```python
from build123d import *

# Parameters (mm, degrees)
F0_W     = 22.7
F0_H     = 42
F1_DEPTH = 13.8
F3_DEPTH = 8.5
F5_DEPTH = 45.1
F7_DEPTH = 3


with BuildPart() as f1:
    # F0 (on Front) → F1 (new body)
    with BuildSketch(Plane.XZ):
        with Locations((0, -9.8)):
            Rectangle(F0_W, F0_H)
    extrude(amount=-F1_DEPTH)

    # F2 (on face) → F3 (join)
    with BuildSketch(Plane.XZ):
        with BuildLine():
            Line((1.966596, 1.85), (-1.966596, 1.85))
            ThreePointArc((-1.966596, 1.85), (-2.7, 0), (-1.966596, -1.85))
            Line((-1.966596, -1.85), (1.966596, -1.85))
            ThreePointArc((1.966596, -1.85), (2.7, 0), (1.966596, 1.85))
        make_face()
    extrude(amount=F3_DEPTH)

    # F4 (on face) → F5 (join)
    with BuildSketch(Plane.XZ):
        with BuildLine():
            Line((7.168159, -13.2), (-7.168159, -13.2))
            ThreePointArc((-7.168159, -13.2), (-11.35, -22), (-7.168159, -30.8))
            Line((-7.168159, -30.8), (7.168159, -30.8))
            ThreePointArc((7.168159, -30.8), (11.35, -22), (7.168159, -13.2))
        make_face()
    extrude(amount=-F5_DEPTH)

    # F6 (on Right) → F7 (join, symmetric)
    with BuildSketch(Plane.YZ):
        Polygon((21.067004, -7.2), (13.8, -7.2), (13.8, -36.8), (21.067004, -36.8), (21.067004, -32.191654), (45.1, -32.191654), (45.1, -11.808346), (21.067004, -11.808346), align=None)
    extrude(amount=F7_DEPTH, both=True)


solid = f1.part
```
CAD build for the part. Positions are in the model's coordinates, mm. A direction names the side the tool comes from. Coordinates: 2 decimals unless noted, no trailing zeros. Order: outer loops, then holes, each group sorted by start corner. A loop starts at its lowest first (then second) coordinate and runs counter-clockwise, first axis right, second up. Notation, with made-up numbers: M -25.5,24 L 17.5,24 A12 cw 17.5,28 Z; hole C 64.25,20.25 d7. An arc over 180 degrees is marked long. Write each question's results on one line, items separated by ' | '. Start each with the question number.
Q1. Which spindle directions (+Z, -Z, +X, -X, +Y, -Y) get a long thin tool onto all of the face, cutting with end or side? Do faces 1 (the flat face through (0, 17, -7.2)), 2 (the flat face through (3, 22, -12)), 3 (the flat face through (-3, 22, -12)). Say none if no direction does.
Q2. Cut at C-C (y = 28.5). List the corners of the cut face in (x, z).
Q3. Cut at A-A (x = 1). List the corners of the cut face in (y, z).
Q4. Cut at B-B (z = -9.5). List the corners of the cut face in (x, y).
Q5. Flat gauge pins, fed straight in: P1, Ø6, axis at x = 3, y = 16.5, coming from the +Z side; P2, Ø1, axis at x = -2, z = -11.5, coming from the -Y side; P3, Ø3.5, axis at x = 1, z = -9.5, coming from the +Y side; P4, Ø5, axis at x = -1.5, y = 26.5, coming from the -Z side. Where does each tip first touch, or does it go through?
Q6. Drill centre lines: probe 1 along Z at (x, y) = (1.5, -4); probe 2 along Y at (x, z) = (7.5, -19); probe 3 along Z at (x, y) = (8.5, 10). Where is each one in solid material? Low to high. Write a range as from..to.
Q7. Cut at D-D (y = 16.5). List the corners of the cut face in (x, z).
Found:
1) face 1: +Z, +X, -X, +Y | face 2: +Z, +X, +Y | face 3: +Z, -X, +Y
2) outline: M -7.17,-30.8 L -3,-30.8 L -3,-32.19 L 3,-32.19 L 3,-30.8 L 7.17,-30.8 A11.35 ccw 7.17,-13.2 L 3,-13.2 L 3,-11.81 L -3,-11.81 L -3,-13.2 L -7.17,-13.2 A11.35 ccw Z
3) outline: M -8.5,-1.85 L 0,-1.85 L 0,-30.8 L 13.8,-30.8 L 13.8,-36.8 L 21.07,-36.8 L 21.07,-32.19 L 45.1,-32.19 L 45.1,-11.81 L 21.07,-11.81 L 21.07,-7.2 L 13.8,-7.2 L 13.8,11.2 L 0,11.2 L 0,1.85 L -8.5,1.85 Z
4) outline: M -11.35,0 L 11.35,0 L 11.35,13.8 L 3,13.8 L 3,21.07 L -3,21.07 L -3,13.8 L -11.35,13.8 Z
5) P1: z = 11.2 | P2: y = 0 | P3: y = 21.07 | P4: z = -32.19
6) probe 1: -1.85..1.85 | probe 2: 0..45.1 | probe 3: -30.8..11.2
7) outline: M -7.17,-30.8 L -3,-30.8 L -3,-36.8 L 3,-36.8 L 3,-30.8 L 7.17,-30.8 A11.35 ccw 7.17,-13.2 L 3,-13.2 L 3,-7.2 L -3,-7.2 L -3,-13.2 L -7.17,-13.2 A11.35 ccw Z
